```python
from build123d import *

# Parameters (mm, degrees)
FILLET1_R          = 10
SKETCH2_R          = 3.175
CUT_EXTRUDE1_DEPTH = 10


with BuildPart() as part:
    # Sketch1 → Revolve1 (revolve)
    with BuildSketch(Plane(origin=(0, 0, 0), x_dir=(1, 0, 0), z_dir=(0, 1, 0)), mode=Mode.PRIVATE) as revolve1_sk:
        Polygon((-27, 157.5), (-27, 15), (-13, 15), (-13, 24.765749007), (-7, 24.765749007), (-7, 15), (0, 15), (0, 0), (-119, 0), (-119, 47), (-97, 47), (-97, 63.5), (-90.65, 63.5), (-90.65, 157.5), align=None)
    revolve(revolve1_sk.sketch.rotate(Axis((-119, 0, 0), (1, 0, 0)), 180), axis=Axis((-119, 0, 0), (1, 0, 0)))

    # Fillet1
    fillet1_edges = [part.edges().sort_by_distance(p)[0] for p in [
        (-27, 0, -157.5),
        (-90.65, 0, -157.5),
    ]]
    fillet(fillet1_edges, radius=FILLET1_R)

    # Sketch2 → Cut-Extrude1 (cut)
    with BuildSketch(Plane.ZY.offset(97)):
        with Locations((0, 58)):
            Circle(SKETCH2_R)
        with Locations((50.229473419, 29)):
            Circle(SKETCH2_R)
        with Locations((50.229473419, -29)):
            Circle(SKETCH2_R)
        with Locations((0, -58)):
            Circle(SKETCH2_R)
        with Locations((-50.22947342, -29)):
            Circle(SKETCH2_R)
        with Locations((-50.229473419, 29)):
            Circle(SKETCH2_R)
    extrude(amount=-CUT_EXTRUDE1_DEPTH, mode=Mode.SUBTRACT)


solid = part.part
```
Work out the finished part from the listing and answer in its coordinate system (mm). A direction names the side the tool comes from. Give positions to 0.01 mm unless a question says otherwise; leave off trailing zeros. Write each loop counter-clockwise with the first axis right and the second up, starting at its lowest first coordinate (ties: lowest second). Pieces come first, ordered by that corner, then holes.
(1) Straight lines are drawn through the part: line 1 (Y direction, x = -93.25, z = 0) (3 decimals); line 2 (X direction, y = -7, z = -13.5); line 3 (X direction, y = -41, z = 30.5). For each, find the intervals that lie inside material, in ascending order.
Final values:
line 1: y = -63.5 to -61.175, -54.825 to 54.825, 61.175 to 63.5
line 2: x = -119 to -27, -13 to -7
line 3: x = -97 to -27
(2) The part is cut by section B-B on x = -18.5. Write down the section's boundary in (y, z).
Final values:
outline: circle Ø30 at (0, 0)
(3) Flat-ended cylindrical pins translate along their axes: pin 1 Ø12 at (x, y) = (-85.5, -49) entering from +Z; pin 2 Ø5 at (y, z) = (102.5, -89) entering from -X; pin 3 Ø1 at (x, y) = (-51, 87) entering from -Z. Find the tip coordinate at first contact, or state that the pin passes through.
Final values:
pin 1: stops at z = 151.11
pin 2: stops at x = -90.65
pin 3: stops at z = -131.62
(4) The part is cut by section A-A on y = 0. Write down the section's boundary in (x, z), plus the area to 3 significant figures.
Final values:
outline: (-119, -47) - (-97, -47) - (-97, -63.5) - (-90.65, -63.5) - (-90.65, -147.5) arc R10 ccw to (-80.65, -157.5) - (-37, -157.5) arc R10 ccw to (-27, -147.5) - (-27, -15) - (-13, -15) - (-13, -24.77) - (-7, -24.77) - (-7, -15) - (0, -15) - (0, 15) - (-7, 15) - (-7, 24.77) - (-13, 24.77) - (-13, 15) - (-27, 15) - (-27, 147.5) arc R10 ccw to (-37, 157.5) - (-80.65, 157.5) arc R10 ccw to (-90.65, 147.5) - (-90.65, 63.5) - (-97, 63.5) - (-97, 47) - (-119, 47) - close
area: 23,800 mm2
(5) Which of the six approach directions +Z, -Z, +X, -X, +Y, -Y give full straight-line access (tool end or side, diameter ignored) to faces 1 (the cylindrical face through (-107.85, -46.6, -6.12)), 2 (the flat face through (-13, 11, -11)), 3 (the flat face through (-119, -1, 1)), 4 (the flat face through (-7, 11, 11)), 5 (the flat face through (0, 0, 0))?
Final values:
face 1: -X
face 2: none
face 3: +Z, -Z, -X, +Y, -Y
face 4: +X
face 5: +Z, -Z, +X, +Y, -Y
(6) The part is cut by section C-C on x = -104. Write down the section's boundary in (y, z), plus the area to 3 significant figures.
Final values:
outline: circle Ø94 at (0, 0)
area: 6,940 mm2
